Study the drawing (mm; zero at the part's minimum x, y, z) and answer. A direction names the side the tool comes from. Give positions to 0.01 mm unless a question says otherwise; leave off trailing zeros. Loops run counter-clockwise (first coordinate to the right, second up) from the corner with the lowest first, then second, coordinate; pieces in that order, holes last. Notation, with made-up numbers: (84, 69) - (124, 69) arc R7 cw to (124, 75) - close; hole circle Ø1 at (56.5, 79). An arc over 180 degrees is marked (long way). Answer in a Markdown table with one row per item. Add a question column.
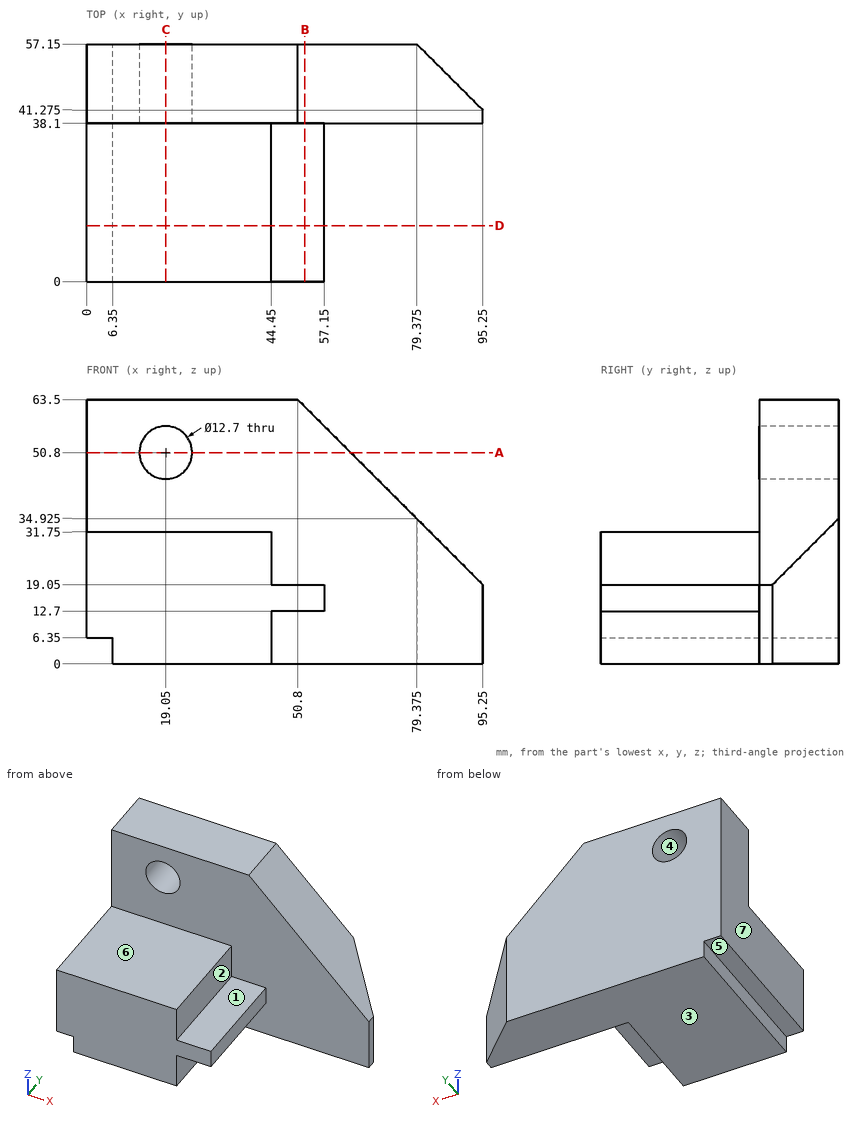
(1) Find the intervals of material crossed by line 1 along Z through (x, y) = (19.05, 49.75); line 2 along Y through (x, z) = (51.5, 44); line 3 along X through (y, z) = (42.5, 48), in increasing order. Write a range as [from, to].
(2) A cutting plane is placed at D-D on y = 13.5. Determine the outline of the cut face in (x, z), plus the area to 3 significant figures.
(3) A tool of negligible diameter and unlimited length cuts with its end or side. For the marked faces 5, 6 and 7, from which of +Z, -Z, +X, -X, +Y, -Y can it reach the whole face along a straight path? Write none if from no direction.
(4) The mould has two halves that part along Z. Classify the marked faces 1, 2, 3 and 4: pulls with the +Z half, pulls with the -Z half, needs draft (parallel to the pull), parting line crosses it, or undercut.
(5) A cutting plane is placed at C-C on x = 19.05. Determine the outline of the cut face in (y, z).
(6) A cutting plane is placed at A-A on z = 50.8. Determine the outline of the cut face in (x, y).
(7) A cutting plane is placed at B-B on x = 52.5. Determine the outline of the cut face in (y, z).
(8) Given pin 1 Ø7 at (y, z) = (22, 2.5) entering from -X; pin 2 Ø1.5 at (y, z) = (44, 28) entering from -X; pin 3 Ø1.9 at (y, z) = (26, 15) entering from +X; pin 4 Ø6.5 at (x, y) = (50.5, 20) entering from -Z, each flat-ended and moving along its own axis, determine where each tip first touches the part or whether it passes through.
Evaluation:
| question | item | result |
|---|---|---|
| 1 | line 1 | z = [0, 44.45], [57.15, 63.5] |
| 1 | line 2 | y = [38.1, 57.15] |
| 1 | line 3 | x = [0, 13.35], [24.75, 66.3] |
| 2 | outline | (0, 6.35) - (6.35, 6.35) - (6.35, 0) - (44.45, 0) - (44.45, 12.7) - (57.15, 12.7) - (57.15, 19.05) - (44.45, 19.05) - (44.45, 31.75) - (0, 31.75) - close |
| 2 | area | 1,450 mm² |
| 3 | face 5 | -Z, -X, +Y, -Y |
| 3 | face 6 | +Z, +X, -X, -Y |
| 3 | face 7 | +Z, -Z, -X, +Y, -Y |
| 4 | face 1 | pulls with the +Z half |
| 4 | face 2 | needs draft |
| 4 | face 3 | pulls with the -Z half |
| 4 | face 4 | undercut |
| 5 | outline | (0, 0) - (57.15, 0) - (57.15, 44.45) - (38.1, 44.45) - (38.1, 31.75) - (0, 31.75) - close; (38.1, 57.15) - (57.15, 57.15) - (57.15, 63.5) - (38.1, 63.5) - close |
| 6 | outline | (0, 38.1) - (12.7, 38.1) - (12.7, 57.15) - (0, 57.15) - close; (25.4, 38.1) - (63.5, 38.1) - (63.5, 57.15) - (25.4, 57.15) - close |
| 7 | outline | (0, 12.7) - (38.1, 12.7) - (38.1, 0) - (57.15, 0) - (57.15, 61.8) - (38.1, 61.8) - (38.1, 19.05) - (0, 19.05) - close |
| 8 | pin 1 | stops at x = 6.35 |
| 8 | pin 2 | stops at x = 0 |
| 8 | pin 3 | stops at x = 57.15 |
| 8 | pin 4 | stops at z = 12.7 |
